Source: CAD feature listing. Evaluate the final solid. Frame: model axes, mm. A direction names the side the tool comes from. Coordinates: 2 decimals unless noted, no trailing zeros. Write each loop counter-clockwise with the first axis right and the second up, starting at its lowest first coordinate (ties: lowest second). Pieces come first, ordered by that corner, then holes. Notation, with made-up numbers: M 89,25 L 145,25 A16 cw 145,40 Z; hole C 51.5,83.25 d5. An arc over 180 degrees is marked long. Write item = value, one per line. Start each with the question number.
1. Access query for faces 4 (the face through (-48, 20, 40)), 5 (the face through (0, 33, 38)), 6 (the face through (-48, 5, 0)), 7 (the face through (-45, 17, 1)), 8 (the face through (-11, 25, -48)). Directions: +Z, -Z, +X, -X, +Y, -Y. A direction counts if a zero-diameter tool reaches every point of the face in a straight line with its end or side. Return the directions, or none.
2. Pin query (flat end, axial travel): pin 1 Ø6 at (x, z) = (17.5, -24) entering from -Y; pin 2 Ø3 at (x, z) = (-47.5, 46) entering from -Y. Return the tip coordinate at first contact, or that it passes through.
3. Section query D-D (x = 2). Output: boundary loops of the cut face in (y, z), then the cut area to 3 significant figures.
4. Section query B-B (z = -11). Output: boundary loops of the cut face in (x, y), then the cut area to 3 significant figures.
5. Pull-direction query (X, two-part tool) for faces 1 (the face through (-1, 20, -50)), 2 (the face through (41, 33, -22)), 3 (the face through (-50, 20, 1)); classes: pulls with the +X half, pulls with the -X half, needs draft (parallel to the pull), parting line crosses it, or undercut.
6. Section query A-A (x = 41). Output: boundary loops of the cut face in (y, z), then the cut area to 3 significant figures.
7. Line query: line 1 along Z through (x, y) = (47.5, 8.5); line 2 along X through (y, z) = (6.15, 46); line 3 along X through (y, z) = (33.5, -3.5). Output: solid intervals per line, ascending.
8. Section query C-C (y = 13.25). Output: boundary loops of the cut face in (x, z).
```python
from build123d import *

# Parameters (mm, degrees)
SKETCH1_W                 = 100
SKETCH1_H                 = 100
BOSS_EXTRUDE1_DEPTH       = 30
SHELL2_T                  = -5
SKETCH2_W                 = 100
SKETCH2_H                 = 100
BOSS_EXTRUDE2_DEPTH       = 5
SKETCH3_W                 = 12
SKETCH3_H                 = 12
SKETCH3_W_2               = 36
SKETCH3_H_2               = 32
SKETCH3_W_3               = 8
SKETCH3_H_3               = 20
CUT_EXTRUDE1_DEPTH        = 5
SKETCH5_W                 = 10
SKETCH5_H                 = 10
CUT_EXTRUDE2_DEPTH        = 5
SKETCH6_W                 = 29
SKETCH6_H                 = 10
CUT_EXTRUDE3_DEPTH        = 5
SKETCH8_W                 = 100
SKETCH8_H                 = 100
CUT_EXTRUDE4_DEPTH        = 5
F_4_0MM_DOWEL_HOLE1_D     = 4
F_4_0MM_DOWEL_HOLE1_DEPTH = 5
F_4_0MM_DOWEL_HOLE1_TIP   = 1.201721238


with BuildPart() as part:
    # Sketch1 → Boss-Extrude1 (new body)
    with BuildSketch(Plane(origin=(0, 0, 0), x_dir=(1, 0, 0), z_dir=(0, 1, 0))):
        Rectangle(SKETCH1_W, SKETCH1_H)
    extrude(amount=BOSS_EXTRUDE1_DEPTH)

    # Shell2
    shell2_openings = [part.faces().sort_by_distance(p)[0] for p in [
        (0, 30, 0),
    ]]
    offset(amount=SHELL2_T, openings=shell2_openings, kind=Kind.INTERSECTION)

    # Sketch2 → Boss-Extrude2 (add)
    with BuildSketch(Plane(origin=(0, 30, 0), x_dir=(1, 0, 0), z_dir=(0, 1, 0))):
        Rectangle(SKETCH2_W, SKETCH2_H)
    extrude(amount=BOSS_EXTRUDE2_DEPTH)

    # Sketch3 → Cut-Extrude1 (cut)
    with BuildSketch(Plane(origin=(0, 35, 0), x_dir=(1, 0, 0), z_dir=(0, 1, 0))):
        with Locations((-14, -32)):
            Rectangle(SKETCH3_W, SKETCH3_H)
        with Locations((0, -32)):
            Rectangle(SKETCH3_W, SKETCH3_H)
        with Locations((14, -32)):
            Rectangle(SKETCH3_W, SKETCH3_H)
        with Locations((0, 12)):
            Rectangle(SKETCH3_W_2, SKETCH3_H_2)
        with Locations((41, 12)):
            Rectangle(SKETCH3_W_3, SKETCH3_H_3)
    extrude(amount=-CUT_EXTRUDE1_DEPTH, mode=Mode.SUBTRACT)

    # Sketch5 → Cut-Extrude2 (cut)
    with BuildSketch(Plane.ZY.offset(50)):
        with Locations((40, 25)):
            Rectangle(SKETCH5_W, SKETCH5_H)
    extrude(amount=-CUT_EXTRUDE2_DEPTH, mode=Mode.SUBTRACT)

    # Sketch6 → Cut-Extrude3 (cut)
    with BuildSketch(Plane(origin=(0, 0, -50), x_dir=(-1, 0, 0), z_dir=(0, 0, -1))):
        with Locations((25.5, 25)):
            Rectangle(SKETCH6_W, SKETCH6_H)
    extrude(amount=-CUT_EXTRUDE3_DEPTH, mode=Mode.SUBTRACT)

    # Sketch8 → Cut-Extrude4 (cut)
    with BuildSketch(Plane.XZ):
        Rectangle(SKETCH8_W, SKETCH8_H)
    extrude(amount=-CUT_EXTRUDE4_DEPTH, mode=Mode.SUBTRACT)

    # Ø4.0mm Dowel Hole1
    with Locations(Plane(origin=(-47.5, 5, 46), x_dir=(0, 0, -1), z_dir=(0, -1, 0))):
        with Locations((0, 0), (0, 95), (92, 95), (92, 0)):
            Hole(F_4_0MM_DOWEL_HOLE1_D / 2, depth=F_4_0MM_DOWEL_HOLE1_DEPTH)
            with Locations((0, 0, -(F_4_0MM_DOWEL_HOLE1_DEPTH + F_4_0MM_DOWEL_HOLE1_TIP / 2))):  # 118° drill point
                Cone(0, F_4_0MM_DOWEL_HOLE1_D / 2, F_4_0MM_DOWEL_HOLE1_TIP, mode=Mode.SUBTRACT)


solid = part.part
```
Results are:
q1.face_4 = -X
q1.face_5 = +Y, -Y
q1.face_6 = +Z, -Z, +X, -X, -Y
q1.face_7 = -Y
q1.face_8 = -Z
q2.pin_1 = 30
q2.pin_2 = 10.3
q3.outline = M 5,-50 L 35,-50 L 35,-28 L 30,-28 L 30,-45 L 5,-45 Z; M 5,45 L 30,45 L 30,38 L 35,38 L 35,50 L 5,50 Z; M 30,4 L 35,4 L 35,26 L 30,26 Z
q3.area = 530 mm^2
q4.outline = M -50,5 L -45,5 L -45,30 L -18,30 L -18,35 L -50,35 Z; M 18,30 L 37,30 L 37,35 L 18,35 Z; M 45,5 L 50,5 L 50,35 L 45,35 Z
q4.area = 530 mm^2
q5.face_1 = needs draft
q5.face_2 = undercut
q5.face_3 = pulls with the -X half
q6.outline = M 5,-50 L 35,-50 L 35,-22 L 30,-22 L 30,-45 L 5,-45 Z; M 5,45 L 30,45 L 30,-2 L 35,-2 L 35,50 L 5,50 Z
q6.area = 650 mm^2
q7.line_1 = -50 to -48, -44 to 44, 48 to 50
q7.line_2 = -50 to -49.5, -45.5 to 45.5, 49.5 to 50
q7.line_3 = -50 to -18, 18 to 37, 45 to 50
q8.outline = M -50,-50 L 50,-50 L 50,50 L -50,50 Z; hole M -45,-45 L 45,-45 L 45,45 L -45,45 Z
